Verification items for the finished model (mm, model axes). Face numbers are marked on the shaded views. Coordinates: 2 decimals unless noted, no trailing zeros. Order: outer loops, then holes, each group sorted by start corner. A loop starts at its lowest first (then second) coordinate and runs counter-clockwise, first axis right, second up. Notation, with made-up numbers: (1, 60.5) -> (33, 60.5) arc R31 cw to (33, 93.5) -> close; hole circle Ø9 at (17, 86.25). An arc over 180 degrees is marked (long way). Use CSV: the item, a comma, the result in double quotes. Start each with the question number.
1) Go/stop test with flat-tipped pins: pin 1 (4.5 mm diameter, centred on x = -842.5, z = -3, fed in from -Y); pin 2 (3 mm diameter, centred on x = -727.5, z = -1.5, fed in from -Y); pin 3 (4.5 mm diameter, centred on x = -838.5, z = -1.5, fed in from +Y). Record where each tip stops, or that it passes through.
2) Sectioned sample at C-C on y = 45.5. Record the boundary of the cut face in (x, z), then the cut area to 3 significant figures.
3) Sectioned sample at B-B on x = -420. Record the boundary of the cut face in (y, z), then the cut area to 3 significant figures.
4) Scan lines: line 1 along X through (y, z) = (2.95, 20); line 2 along Y through (x, z) = (138.5, 37); line 3 along Z through (x, y) = (-600, 76.5). Record each from-to range of solid material in increasing order.
5) Release check for a two-part mould opening along Y. For the marked faces 1 and 2 record: released by +Y, released by -Y, zero draft, split by the parting line, or undercut.
6) Sectioned sample at A-A on z = 20. Record the boundary of the cut face in (x, y), then the cut area to 3 significant figures.
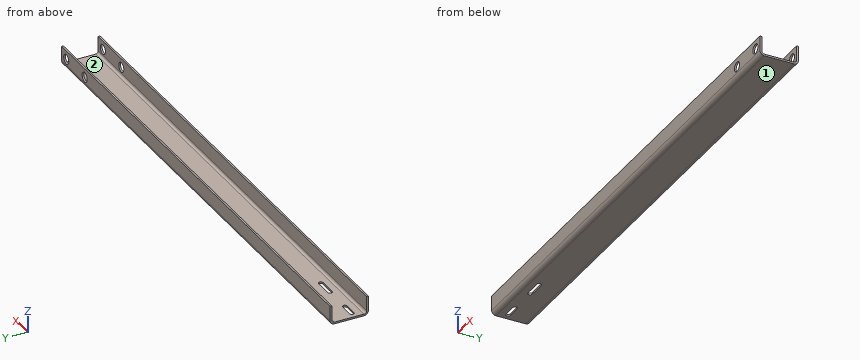
from build123d import *

# Parameters (mm, degrees)
SKETCH1_W                    = 1165
SKETCH1_H                    = 88
BASE_FLANGE1_DEPTH           = 4
EDGE_FLANGE1_STRIP_W         = 28
EDGE_FLANGE1_STRIP_H         = 4
EDGE_FLANGE1_STRIP_CUT_DEPTH = 1165
EDGE_FLANGE1_DEPTH           = 1165
EDGE_FLANGE2_STRIP_W         = 28
EDGE_FLANGE2_STRIP_H         = 4
EDGE_FLANGE2_STRIP_CUT_DEPTH = 1165
EDGE_FLANGE2_DEPTH           = 1165
CUT_EXTRUDE1_DEPTH           = 871.900176512
CUT_EXTRUDE1_DEPTH_BACK      = 871.900176512
SKETCH12_R                   = 11
CUT_EXTRUDE2_DEPTH           = 872.093059006


# Sheet-metal steps are written as plain solids
with BuildPart() as part:
    # Sketch1 → Base-Flange1 (new body)
    with BuildSketch(Plane.XY):
        with Locations((-283.018987342, 44)):
            Rectangle(SKETCH1_W, SKETCH1_H)
    extrude(amount=-BASE_FLANGE1_DEPTH)

    # Edge-Flange1 strip (across the edge) → Edge-Flange1 strip cut (cut)
    with BuildSketch(Plane(origin=(299.481012658, 88, 0), x_dir=(0, -1, 0), z_dir=(-1, 0, 0))):
        with Locations((-4, -2)):
            Rectangle(EDGE_FLANGE1_STRIP_W, EDGE_FLANGE1_STRIP_H)
    extrude(amount=EDGE_FLANGE1_STRIP_CUT_DEPTH, mode=Mode.SUBTRACT)

    # Edge-Flange1 section (across the edge) → Edge-Flange1 (add)
    with BuildSketch(Plane(origin=(299.481012658, 88, 0), x_dir=(0, -1, 0), z_dir=(-1, 0, 0))):
        with BuildLine():
            Line((0, 6), (0, 40))
            Line((0, 40), (4, 40))
            Line((4, 40), (4, 6))
            ThreePointArc((4, 6), (5.757359313, 1.757359313), (10, 0))
            Line((10, 0), (10, -4))
            ThreePointArc((10, -4), (2.928932188, -1.071067812), (0, 6))
        make_face()
    extrude(amount=EDGE_FLANGE1_DEPTH)

    # Edge-Flange2 strip (across the edge) → Edge-Flange2 strip cut (cut)
    with BuildSketch(Plane.YZ.offset(-865.518987342)):
        with Locations((-4, -2)):
            Rectangle(EDGE_FLANGE2_STRIP_W, EDGE_FLANGE2_STRIP_H)
    extrude(amount=EDGE_FLANGE2_STRIP_CUT_DEPTH, mode=Mode.SUBTRACT)

    # Edge-Flange2 section (across the edge) → Edge-Flange2 (add)
    with BuildSketch(Plane.YZ.offset(-865.518987342)):
        with BuildLine():
            Line((0, 6), (0, 40))
            Line((0, 40), (4, 40))
            Line((4, 40), (4, 6))
            ThreePointArc((4, 6), (5.757359313, 1.757359313), (10, 0))
            Line((10, 0), (10, -4))
            ThreePointArc((10, -4), (2.928932188, -1.071067812), (0, 6))
        make_face()
    extrude(amount=EDGE_FLANGE2_DEPTH)

    # Sketch12 → Cut-Extrude1 (cut, two sides: drawn at the far end of the back side and taken through both)
    with BuildSketch(Plane.XZ.offset(-CUT_EXTRUDE1_DEPTH_BACK)):
        with Locations(Location((279.481012658, 20, 0), (0, 0, 270))):
            Circle(SKETCH12_R)
        with Locations(Location((199.481012658, 20, 0), (0, 0, 270))):
            Circle(SKETCH12_R)
    extrude(amount=CUT_EXTRUDE1_DEPTH + CUT_EXTRUDE1_DEPTH_BACK, mode=Mode.SUBTRACT)

    # Sketch13 → Cut-Extrude2 (cut, through all)
    with BuildSketch(Plane(origin=(0, 0, -4), x_dir=(-1, 0, 0), z_dir=(0, 0, -1))):
        with BuildLine():
            Line((850.518987342, 25), (820.518987342, 25))
            ThreePointArc((820.518987342, 25), (815.518987342, 30), (820.518987342, 35))
            Line((820.518987342, 35), (850.518987342, 35))
            ThreePointArc((850.518987342, 35), (855.518987342, 30), (850.518987342, 25))
        make_face()
        with BuildLine():
            Line((755.518987342, 25), (715.518987342, 25))
            ThreePointArc((715.518987342, 25), (710.518987342, 30), (715.518987342, 35))
            Line((715.518987342, 35), (755.518987342, 35))
            ThreePointArc((755.518987342, 35), (760.518987342, 30), (755.518987342, 25))
        make_face()
    extrude(amount=-CUT_EXTRUDE2_DEPTH, mode=Mode.SUBTRACT)


solid = part.part
Answers follow:
1,pin 1,"stops at y = 2.62"
1,pin 2,"stops at y = 2"
1,pin 3,"stops at y = 86.51"
2,outline,"(-865.52, -4) -> (299.48, -4) -> (299.48, 0) -> (-865.52, 0) -> close"
2,area,"4,660 mm²"
3,outline,"(0, 6) arc R10 ccw to (10, -4) -> (78, -4) arc R10 ccw to (88, 6) -> (88, 40) -> (84, 40) -> (84, 6) arc R6 cw to (78, 0) -> (10, 0) arc R6 cw to (4, 6) -> (4, 40) -> (0, 40) -> close"
3,area,"645 mm²"
4,line 1,"x = -865.52 to 188.48, 210.48 to 268.48, 290.48 to 299.48"
4,line 2,"y = 0 to 4, 84 to 88"
4,line 3,"z = -4 to 0"
5,face 1,"zero draft"
5,face 2,"undercut"
6,outline,"(-865.52, 0) -> (188.48, 0) -> (188.48, 4) -> (-865.52, 4) -> close; (-865.52, 84) -> (188.48, 84) -> (188.48, 88) -> (-865.52, 88) -> close; (210.48, 0) -> (268.48, 0) -> (268.48, 4) -> (210.48, 4) -> close; (210.48, 84) -> (268.48, 84) -> (268.48, 88) -> (210.48, 88) -> close; (290.48, 0) -> (299.48, 0) -> (299.48, 4) -> (290.48, 4) -> close; (290.48, 84) -> (299.48, 84) -> (299.48, 88) -> (290.48, 88) -> close"
6,area,"8,970 mm²"
